Geometry: final body of the model. Coordinates: model frame, mm. Face numbers are marked on the shaded views. A direction names the side the tool comes from. Round coordinates to 2 decimals unless told otherwise and drop trailing zeros. Loops run counter-clockwise (first coordinate to the right, second up) from the corner with the lowest first, then second, coordinate; pieces in that order, holes last. Notation, with made-up numbers: (18, 58.25) - (23, 58.25) arc R30 cw to (23, 85.25) - close; hole circle Ø6 at (45, 29.25). An arc over 180 degrees is marked (long way). Write item = value, one per line. Start each with the question number.
Item 1: Section C-C (z = -23.5). Return loops of the section in (x, y), plus the area to 3 significant figures.
Item 2: Access query for the marked faces 1 and 2. Directions: +Z, -Z, +X, -X, +Y, -Y. A direction counts if a zero-diameter tool reaches every point of the face in a straight line with its end or side. Return the directions, or none.
Item 3: Section B-B (z = -18.5). Return loops of the section in (x, y).
Item 4: Draft query along X for the marked faces 3 and 4. Return one class per face: pulls with the +X half, pulls with the -X half, needs draft (parallel to the pull), parting line crosses it, or undercut.
Item 5: Section A-A (x = 0). Return loops of the section in (y, z), plus the area to 3 significant figures.
Item 6: Line query: line 1 (Z direction, x = -4, y = -2.5); line 2 (X direction, y = -0.25, z = -3); line 3 (Z direction, x = 1, y = -1). Output: solid intervals per line, ascending. Write a range as from..to.
Item 7: First-contact query: pin 1 (2 mm diameter, centred on x = 3, z = -18, fed in from -Y); pin 2 (5 mm diameter, centred on y = 4, z = -13, fed in from -X); pin 3 (5 mm diameter, centred on x = 0, z = -16, fed in from +Y). Flat tips, straight axial feed; report the tip coordinate or a pass-through.
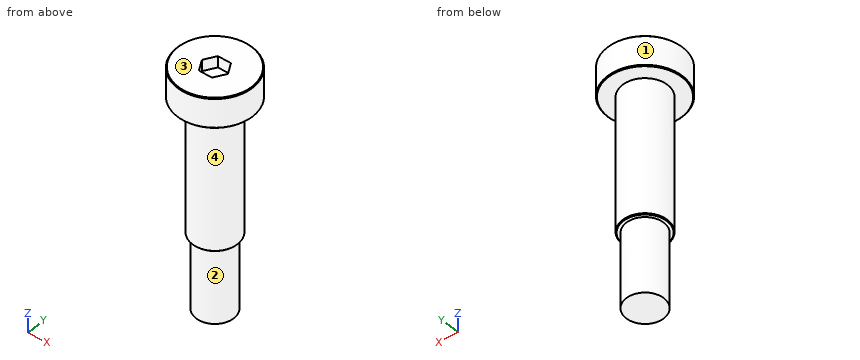
from build123d import *

# Parameters (mm, degrees)
SKETCH_1_R          = 5
EXTRUDE_1_DEPTH     = 4
SKETCH_2_R          = 3
EXTRUDE_2_DEPTH     = 18
SKETCH_3_R          = 2.5
EXTRUDE_3_DEPTH     = 10
CHAMFER_1_SIZE      = 0.1
CUT_EXTRUDE_1_DEPTH = 1.5


with BuildPart() as part:
    # 草图1 → 凸台-拉伸1 (new body)
    with BuildSketch(Plane.XY):
        Circle(SKETCH_1_R)
    extrude(amount=-EXTRUDE_1_DEPTH)

    # 草图2 → 凸台-拉伸2 (add)
    with BuildSketch(Plane(origin=(0, 0, -4), x_dir=(-1, 0, 0), z_dir=(0, 0, -1))):
        Circle(SKETCH_2_R)
    extrude(amount=EXTRUDE_2_DEPTH)

    # 草图3 → 凸台-拉伸3 (add)
    with BuildSketch(Plane(origin=(0, 0, -22), x_dir=(-1, 0, 0), z_dir=(0, 0, -1))):
        Circle(SKETCH_3_R)
    extrude(amount=EXTRUDE_3_DEPTH)

    # 倒角1
    chamfer_1_edges = [part.edges().sort_by_distance(p)[0] for p in [
        (-5, 0, 0),
        (-5, 0, -4),
        (3, 0, -22),
    ]]
    chamfer(chamfer_1_edges, length=CHAMFER_1_SIZE)

    # 草图4 → 切除-拉伸1 (cut)
    with BuildSketch(Plane.XY):
        Polygon((1.732050808, 0), (0.866025404, 1.5), (-0.866025404, 1.5), (-1.732050808, 0), (-0.866025404, -1.5), (0.866025404, -1.5), align=None)
    extrude(amount=-CUT_EXTRUDE_1_DEPTH, mode=Mode.SUBTRACT)


solid = part.part
Taken from the geometry:
q1.outline = circle Ø5 at (0, 0)
q1.area = 19.6 mm^2
q2.face_1 = +Z, -Z
q2.face_2 = -Z
q3.outline = circle Ø6 at (0, 0)
q4.face_3 = needs draft
q4.face_4 = parting line crosses it
q5.outline = (-5, -3.9) - (-4.9, -4) - (-3, -4) - (-3, -21.9) - (-2.9, -22) - (-2.5, -22) - (-2.5, -32) - (2.5, -32) - (2.5, -22) - (2.9, -22) - (3, -21.9) - (3, -4) - (4.9, -4) - (5, -3.9) - (5, -0.1) - (4.9, 0) - (1.5, 0) - (1.5, -1.5) - (-1.5, -1.5) - (-1.5, 0) - (-4.9, 0) - (-5, -0.1) - close
q5.area = 193 mm^2
q6.line_1 = -4..0
q6.line_2 = -4.99..4.99
q6.line_3 = -32..-1.5
q7.pin_1 = -2.24
q7.pin_2 = -2.6
q7.pin_3 = 3
